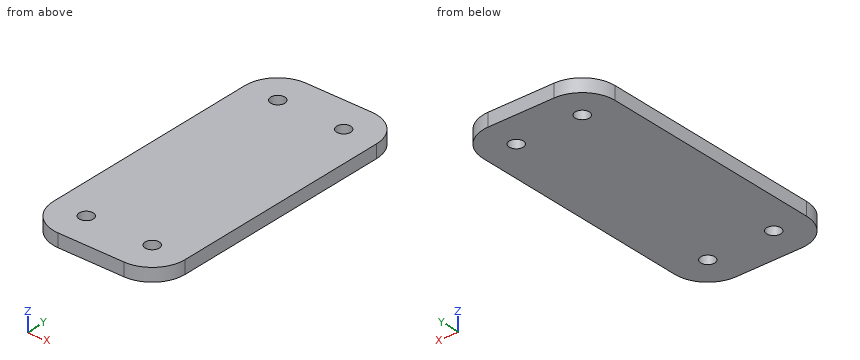
Autodesk Inventor part; units mm, degrees
ref_plane "YZ Plane" through (0, 0, 0) normal (1, 0, 0) x (0, 1, 0)
ref_plane "XZ Plane" through (0, 0, 0) normal (0, 1, 0) x (-1, 0, 0)
ref_plane "XY Plane" through (0, 0, 0) normal (0, 0, 1) x (1, 0, 0)
sketch "スケッチ1" plane through (0, 0, 0) normal (0, 0, 1) x (1, 0, 0)
  circle A0 centre (0, 0) radius 1.6
  circle A1 centre (15, 0) radius 1.6
  circle A2 centre (0, 51) radius 1.6
  circle A3 centre (15, 51) radius 1.6
  line L0 (-7.5, -7.5) -> (22.5, -7.5)
  line L1 (22.5, -7.5) -> (22.5, 58.5)
  line L2 (22.5, 58.5) -> (-7.5, 58.5)
  line L3 (-7.5, 58.5) -> (-7.5, -7.5)
  dimension "d0" = 3.2
  dimension "d1" = 3.2
  dimension "d2" = 3.2
  dimension "d3" = 3.2
  dimension "d4" = 15
  dimension "d5" = 51
  dimension "d6" = 7.5
  dimension "d7" = 7.5
  dimension "d8" = 7.5
  dimension "d9" = 7.5
extrude "押し出し1" add sketch "スケッチ1" along normal blind 3
fillet "フィレット1" radius 7.5 4 edges at (-7.5, 58.5, 1.5) (22.5, 58.5, 1.5) (22.5, -7.5, 1.5) (-7.5, -7.5, 1.5)
sketch "スケッチ2" plane through (0, 0, 3) normal (0, 0, 1) x (1, 0, 0)
  point P0 (0, 0)
properties part number "オムニ_固定具4" material "アルミニウム 6061"
Geometry check sheet. Reference: the model listing, model coordinates, mm. Coordinates: 2 decimals unless noted, no trailing zeros. Loops run counter-clockwise (first coordinate to the right, second up) from the corner with the lowest first, then second, coordinate; pieces in that order, holes last.
Item 1: Thickness scan on line 1 (Y direction, x = 0, z = 1.85); line 2 (X direction, y = 0.5, z = 1.3); line 3 (X direction, y = -2.5, z = 0.3). Record the ranges inside material, lowest first.
Item 2: Sectioned sample at B-B, the plane y = -3. Record the boundary of the cut face in (x, z).
Item 3: Go/stop test with a flat-tipped pin: pin 1 Ø1 at (x, z) = (18.5, 2) entering from +Y. Record where the tip stops, or that it passes through.
Item 4: Sectioned sample at A-A, the plane z = 1.35. Record the boundary of the cut face in (x, y).
Check result:
1. line 1: y = -7.5 to -1.6, 1.6 to 49.4, 52.6 to 58.5
1. line 2: x = -7.5 to -1.52, 1.52 to 13.48, 16.52 to 22.5
1. line 3: x = -7.07 to 22.07
2. outline: (-6.87, 0) - (21.87, 0) - (21.87, 3) - (-6.87, 3) - close
3. pin 1: stops at y = 57.87
4. outline: (-7.5, 0) arc R7.5 ccw to (0, -7.5) - (15, -7.5) arc R7.5 ccw to (22.5, 0) - (22.5, 51) arc R7.5 ccw to (15, 58.5) - (0, 58.5) arc R7.5 ccw to (-7.5, 51) - close; hole circle Ø3.2 at (0, 0); hole circle Ø3.2 at (0, 51); hole circle Ø3.2 at (15, 0); hole circle Ø3.2 at (15, 51)
